Can you work these out from the model? Positions are in its coordinate system, mm. A direction names the side the tool comes from. Round coordinates to 2 decimals unless told otherwise and drop trailing zeros. Loops run counter-clockwise (first coordinate to the right, second up) from the corner with the lowest first, then second, coordinate; pieces in that order, holes last.
(1) I want a section at D-D on x = -106.5. Write out the boundary of the cut face in (y, z), plus the area to 3 significant figures.
(2) Will this pin go through, and if not, where does the flat tip stop? pin 1 Ø10 at (x, y) = (42.5, -83) entering from +Z.
(3) Which directions (+Z, -Z, +X, -X, +Y, -Y) give clear straight access to the entire face, cutting with the end or side of a thin tool? Please do faces 1 (the face through (36, 24, 5)), 2 (the face through (-1, 135, 12)), 3 (the face through (2, 130, 9)).
(4) If I drill on line 1 along X through (y, z) = (135, 4.5); line 2 along Y through (x, z) = (42.5, 5.2), over which ranges is the centre line in solid material (lowest first)?
(5) Thinking about a two-plate mould opening in Y: for faces 4 (the face through (-2, 140, 6)), 5 (the face through (-130, 2, 9)), 6 (the face through (130, -2, 9)), 7 (the face through (140, 2, 6)), which applies, released by +Y, released by -Y, zero draft, split by the parting line, or undercut?
(6) I want a section at A-A on z = 2.25. Write out the boundary of the cut face in (x, y), plus the area to 3 significant figures.
(7) I want a section at B-B on x = 0. Write out the boundary of the cut face in (y, z), plus the area to 3 significant figures.
Autodesk Inventor part; units mm, degrees
ref_plane "YZ Plane" through (0, 0, 0) normal (1, 0, 0) x (0, 1, 0)
ref_plane "XZ Plane" through (0, 0, 0) normal (0, 1, 0) x (-1, 0, 0)
ref_plane "XY Plane" through (0, 0, 0) normal (0, 0, 1) x (1, 0, 0)
sketch "Sketch1" plane through (0, 0, 0) normal (0, 0, 1) x (1, 0, 0)
  line L0 (-140, 140) -> (140, 140)
  line L1 (140, 140) -> (140, -140)
  line L2 (140, -140) -> (-140, -140)
  line L3 (-140, -140) -> (-140, 140)
  point P0 (0, 0)
  point P1 (0, 140)
  point P2 (140, 0)
  dimension "d0" = 280
  dimension "d1" = 280
extrude "Extrusion1" add sketch "Sketch1" along normal blind 6
sketch "Sketch2" plane through (0, 0, 6) normal (0, 0, 1) x (1, 0, 0)
  line L0 (140, 140) -> (-140, 140)
  line L1 (-140, 140) -> (-140, -140)
  line L2 (-140, -140) -> (140, -140)
  line L3 (140, -140) -> (140, 140)
  line L4 (130, 130) -> (-130, 130)
  line L5 (-130, 130) -> (-130, -130)
  line L6 (-130, -130) -> (130, -130)
  line L7 (130, -130) -> (130, 130)
  point P0 (0, 0)
  dimension "d4" = 10
extrude "Extrusion2" add sketch "Sketch2" along normal blind 6
sketch "Sketch3" plane through (0, 0, 12) normal (0, 0, 1) x (1, 0, 0)
  circle A0 centre (-135, -135) radius 2.05
  circle A1 centre (-135, 135) radius 2.05
  line L0 (-135, 135) -> (-135, -135) construction
  line L1 (-140, 140) -> (-140, -140) construction
  line L2 (-140, -140) -> (140, -140) construction
  point P0 (0, 0)
  point P1 (-135, 0)
  point P2 (-140, 0)
  dimension "d7" = 4.1
  dimension "d8" = 4.1
  dimension "d9" = 5
  dimension "d10" = 5
extrude "Extrusion3" cut sketch "Sketch3" against normal up to surface (12 mm away)
mirror "Mirror1" about plane through (0, 0, 0) normal (1, 0, 0) of "Extrusion3"
sketch "Sketch4" plane through (0, 0, 0) normal (0, 0, -1) x (-1, 0, 0)
  line L0 (-52.5, 52.5) -> (52.5, 52.5)
  line L1 (52.5, 52.5) -> (52.5, -52.5)
  line L2 (52.5, -52.5) -> (-52.5, -52.5)
  line L3 (-52.5, -52.5) -> (-52.5, 52.5)
  point P0 (0, 0)
  point P1 (52.5, 0)
  point P2 (0, 52.5)
  dimension "d13" = 105
  dimension "d14" = 105
extrude "Extrusion4" cut sketch "Sketch4" against normal blind 5
sketch "Sketch5" plane through (0, 0, 5) normal (0, 0, -1) x (-1, 0, 0)
  circle A0 centre (0, 0) radius 39
  dimension "d17" = 78
extrude "Extrusion5" cut sketch "Sketch5" against normal blind 5
sketch "Sketch6" plane through (0, 0, 5) normal (0, 0, -1) x (-1, 0, 0)
  circle A0 centre (-42.5, 42.5) radius 2.75
  line L0 (-52.5, 52.5) -> (52.5, 52.5)
  line L1 (-52.5, -52.5) -> (-52.5, 52.5)
  point P0 (0, 0)
  dimension "d27" = 5.5
  dimension "d28" = 10
  dimension "d29" = 10
extrude "Extrusion6" cut sketch "Sketch6" against normal blind 5
pattern_linear "Rectangular Pattern1" count 2 spacing 85 along (0, -1, 0) count 2 spacing 85 along (-1, 0, 0) of "Extrusion6"
properties part number "brain box top"
Filled sheet:
1. outline: (-140, 0) - (140, 0) - (140, 12) - (130, 12) - (130, 6) - (-130, 6) - (-130, 12) - (-140, 12) - close
1. area: 1,800 mm2
2. pin 1: stops at z = 6
3. face 1: -Z
3. face 2: +Z, +X, -X, +Y, -Y
3. face 3: +Z
4. line 1: x = -140 to -137.05, -132.95 to 132.95, 137.05 to 140
4. line 2: y = -140 to -45.25, -39.75 to 39.75, 45.25 to 140
5. face 4: released by +Y
5. face 5: undercut
5. face 6: undercut
5. face 7: zero draft
6. outline: (-140, -140) - (140, -140) - (140, 140) - (-140, 140) - close; hole circle Ø4.1 at (-135, -135); hole circle Ø4.1 at (-135, 135); hole (-52.5, -52.5) - (52.5, -52.5) - (52.5, 52.5) - (-52.5, 52.5) - close; hole circle Ø4.1 at (135, -135); hole circle Ø4.1 at (135, 135)
6. area: 67,300 mm2
7. outline: (-140, 0) - (-52.5, 0) - (-52.5, 5) - (-39, 5) - (-39, 6) - (-130, 6) - (-130, 12) - (-140, 12) - close; (39, 5) - (52.5, 5) - (52.5, 0) - (140, 0) - (140, 12) - (130, 12) - (130, 6) - (39, 6) - close
7. area: 1,200 mm2
